The model under review builds one solid part; all positions refer to its coordinate system, in mm. A direction names the side the tool comes from. Round coordinates to 2 decimals unless told otherwise and drop trailing zeros. Write each loop counter-clockwise with the first axis right and the second up, starting at its lowest first coordinate (ties: lowest second). Pieces come first, ordered by that corner, then holes. Notation, with made-up numbers: (86, 75) -> (144, 75) arc R22 ccw to (144, 92) -> close; hole circle Ø6 at (36.5, 89.5). An arc over 180 degrees is marked (long way). Return JSON: item names as keys, results as strings. Group by question number.
1. Clearance check with flat-ended pins moving along their axes: P1, Ø8, axis at x = 74, y = -81.5, coming from the -Z side; P2, Ø4, axis at x = 68.5, z = -1.5, coming from the +Y side; P3, Ø4, axis at x = -78, z = -1, coming from the -Y side. State where each tip first meets the part, or that it passes through.
2. Mouldability with a two-part tool opening along X and no side actions: class faces 6 (the cylindrical face through (96.48, -30.38, -5.07)), 7 (the flat face through (-114, -4, -2)), 8 (the cylindrical face through (106.15, -0.09, -3.7)) as pulls with the +X half, pulls with the -X half, needs draft (parallel to the pull), parting line crosses it, or undercut.
3. For line 1 along Y through (x, z) = (0, -4.5); line 2 along X through (y, z) = (29, -8.5); line 3 along X through (y, z) = (40, -9), list the stretches that pass through material, from the lowest coordinate up. Write a range as from..to.
4. Tool access review of faces 1 (the flat face through (-4, 114, -2)), 2 (the flat face through (114, -4, -2)), 3 (the flat face through (-4, -114, -2)), 4 (the cylindrical face through (-75.12, -75, -3.7)), 5 (the flat face through (-114, 4, -2)): name each direction out of +Z, -Z, +X, -X, +Y, -Y from which nothing blocks a thin tool from reaching the whole face with its end or side.
5. Take a section at A-A, the plane x = 0. Write out the cut boundary in (y, z).
from build123d import *

# Parameters (mm, degrees)
CUT_EXTRUDE1_DEPTH = 10
CIRPATTERN1_COUNT  = 8


with BuildPart() as part:
    # Sketch2 → Revolve1 (revolve)
    with BuildSketch(Plane(origin=(0, 0, 0), x_dir=(0, 0, -1), z_dir=(1, 0, 0)), mode=Mode.PRIVATE) as revolve1_sk:
        Polygon((0, 121.15), (0, 101.15), (10, 101.15), align=None)
    revolve(revolve1_sk.sketch.rotate(Axis((0, 0, 25.61681186), (0, 0, -1)), 90), axis=Axis((0, 0, 25.61681186), (0, 0, -1)))

    # Sketch3 → Cut-Extrude1 (cut)
    with BuildSketch(Plane.XY):
        with BuildLine():
            Line((-4, 110.15), (-4, 131.372704066))
            Line((-4, 131.372704066), (4, 131.372704066))
            Line((4, 131.372704066), (4, 110.15))
            ThreePointArc((4, 110.15), (0, 106.15), (-4, 110.15))
        make_face()
    cut_extrude1 = extrude(amount=-CUT_EXTRUDE1_DEPTH, mode=Mode.SUBTRACT)

    # CirPattern1: Cut-Extrude1 ×8 about axis
    cirpattern1_axis = Axis((0, 0, 0), (0, 0, 1))
    for i in range(1, CIRPATTERN1_COUNT):
        add(cut_extrude1.rotate(cirpattern1_axis, i * 360 / CIRPATTERN1_COUNT), mode=Mode.SUBTRACT)


solid = part.part
Output:
{
 "1": {"P1": "stops at z = -7.53", "P2": "stops at y = 100.82", "P3": "stops at y = -94.13"},
 "2": {"face 6": "undercut", "face 7": "needs draft", "face 8": "pulls with the +X half"},
 "3": {"line 1": "y = -106.15..-101.15, 101.15..106.15", "line 2": "x = -100.03..-96.9, 96.9..100.03", "line 3": "x = -95.08..-92.9, 92.9..95.08"},
 "4": {"face 1": "+Z, -Z, +Y", "face 2": "+Z, -Z, +X", "face 3": "+Z, -Z, -Y", "face 4": "+Z, -Z", "face 5": "+Z, -Z, -X"},
 "5": {"outline": "(-106.15, -7.5) -> (-101.15, -10) -> (-101.15, 0) -> (-106.15, 0) -> close; (101.15, -10) -> (106.15, -7.5) -> (106.15, 0) -> (101.15, 0) -> close"}
}
